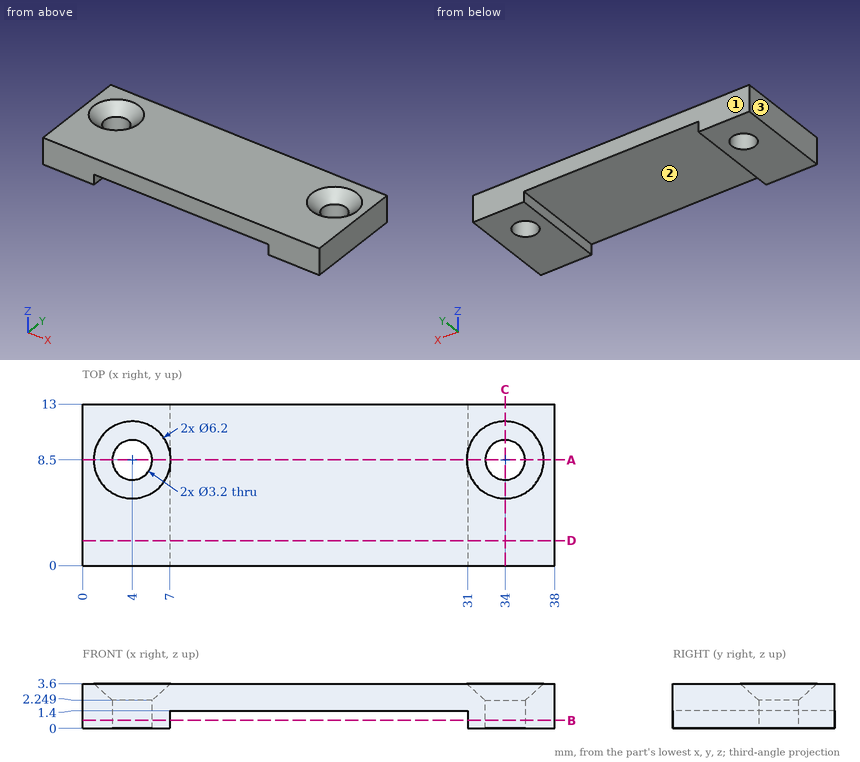
Print and shaded views of the part. All mm, measured from the part's lowest x, y and z. Coordinates: 2 decimals unless noted, no trailing zeros. Order: outer loops, then holes, each group sorted by start corner. A loop starts at its lowest first (then second) coordinate and runs counter-clockwise, first axis right, second up. Notation, with made-up numbers: (8, 47) -> (40, 47) arc R13 cw to (40, 55) -> close; hole circle Ø4 at (24.25, -6). An arc over 180 degrees is marked (long way). Use one line per item in the form item = value. Start each with the question number.
1) Band-saw the part on A-A on y = 8.5. Give the cut face in (x, z).
2) Band-saw the part on B-B on z = 0.65. Give the cut face in (x, y), then the cut area to 3 significant figures.
3) Band-saw the part on D-D on y = 2. Give the cut face in (x, z), then the cut area to 3 significant figures.
4) Pull direction X, two halves, no side cores. Call the marked faces 1, 2 and 3: +X half, -X half, draft (parallel to the pull), parting line (faces both ways), or undercut.
5) Band-saw the part on C-C on x = 34. Give the cut face in (y, z).
6) Drop flat-ended pins along their axis: pin 1 (1.1 mm diameter, centred on y = 4, z = 1, fed in from -X); pin 2 (1.5 mm diameter, centred on x = 12.5, y = 11.5, fed in from -Z); pin 3 (4 mm diameter, centred on x = 4, y = 8.5, fed in from +Z). Give the stop position or say it passes through.
7) Drill centre lines: L1, parallel to Y at x = 34, z = 0.85; L2, parallel to X at y = 8.75, z = 2.1; L3, parallel to X at y = 6.5, z = 0.8. Where is each one in solid material? Low to high. Write a range as [from, to].
Entries:
q1.outline = (0, 0) -> (2.4, 0) -> (2.4, 2.25) -> (0.9, 3.6) -> (0, 3.6) -> close; (5.6, 0) -> (7, 0) -> (7, 1.4) -> (31, 1.4) -> (31, 0) -> (32.4, 0) -> (32.4, 2.25) -> (30.9, 3.6) -> (7.1, 3.6) -> (5.6, 2.25) -> close; (35.6, 0) -> (38, 0) -> (38, 3.6) -> (37.1, 3.6) -> (35.6, 2.25) -> close
q2.outline = (0, 0) -> (7, 0) -> (7, 13) -> (0, 13) -> close; (31, 0) -> (38, 0) -> (38, 13) -> (31, 13) -> close; hole circle Ø3.2 at (4, 8.5); hole circle Ø3.2 at (34, 8.5)
q2.area = 166 mm2
q3.outline = (0, 0) -> (7, 0) -> (7, 1.4) -> (31, 1.4) -> (31, 0) -> (38, 0) -> (38, 3.6) -> (0, 3.6) -> close
q3.area = 103 mm2
q4.face_1 = draft
q4.face_2 = undercut
q4.face_3 = -X half
q5.outline = (0, 0) -> (6.9, 0) -> (6.9, 2.25) -> (5.4, 3.6) -> (0, 3.6) -> close; (10.1, 0) -> (13, 0) -> (13, 3.6) -> (11.6, 3.6) -> (10.1, 2.25) -> close
q6.pin_1 = 0
q6.pin_2 = 1.4
q6.pin_3 = 2.61
q7.L1 = [0, 6.9], [10.1, 13]
q7.L2 = [0, 2.42], [5.58, 32.42], [35.58, 38]
q7.L3 = [0, 7], [31, 38]
